from build123d import *

# Parameters (mm, degrees)
BOSS_EXTRUDE1_DEPTH = 19
SKETCH2_W           = 19
SKETCH2_H           = 80
BOSS_EXTRUDE2_DEPTH = 19
SKETCH3_W           = 19
SKETCH3_H           = 80
BOSS_EXTRUDE3_DEPTH = 19


with BuildPart() as part:
    # Sketch1 → Boss-Extrude1 (new body)
    with BuildSketch(Plane(origin=(0, 0, 0), x_dir=(0, 0, -1), z_dir=(1, 0, 0))):
        with BuildLine():
            Line((-143.772893773, 109.432234432), (-143.772893773, -140.567765568))
            Line((-143.772893773, -140.567765568), (96.227106227, -140.567765568))
            ThreePointArc((96.227106227, -140.567765568), (-42.958076814, -33.985541287), (-143.772893773, 109.432234432))
        make_face()
    extrude(amount=BOSS_EXTRUDE1_DEPTH)

    # Sketch2 → Boss-Extrude2 (add)
    with BuildSketch(Plane.XZ.offset(140.567765568)):
        with Locations((9.5, 23.772893773)):
            Rectangle(SKETCH2_W, SKETCH2_H)
    extrude(amount=BOSS_EXTRUDE2_DEPTH)

    # Sketch3 → Boss-Extrude3 (add)
    with BuildSketch(Plane.XY.offset(143.772893773)):
        with Locations((9.5, -20.567765568)):
            Rectangle(SKETCH3_W, SKETCH3_H)
    extrude(amount=BOSS_EXTRUDE3_DEPTH)


solid = part.part
CAD build for the part. Positions are in the model's coordinates, mm. A direction names the side the tool comes from. Round coordinates to 2 decimals unless told otherwise and drop trailing zeros. Order: outer loops, then holes, each group sorted by start corner. A loop starts at its lowest first (then second) coordinate and runs counter-clockwise, first axis right, second up. Notation, with made-up numbers: (18, 88.5) - (36, 88.5) arc R17 ccw to (36, 96.5) - close; hole circle Ø9 at (68.5, 20). An arc over 180 degrees is marked (long way). Return JSON: item names as keys, results as strings.
(1) Cut at A-A (x = 12.5). Give the cut face in (y, z).
Answer key:
{"outline": "(-159.57, -16.23) - (-140.57, -16.23) - (-140.57, -96.23) arc R577.79 cw to (109.43, 143.77) - (19.43, 143.77) - (19.43, 162.77) - (-60.57, 162.77) - (-60.57, 143.77) - (-140.57, 143.77) - (-140.57, 63.77) - (-159.57, 63.77) - close"}
(2) Tool access for faces 1 (the face through (9, 19.432, 153)), 2 (the face through (9, -140.568, -56)), 3 (the face through (9, -60.568, 153)), 4 (the face through (0, -64, 72)), 5 (the face through (9.37, -35.76, 41.25)): list every direction of +Z, -Z, +X, -X, +Y, -Y with a clear straight run to the whole face (end or side of a thin tool).
Answer key:
{"face 1": "+Z, +X, -X, +Y", "face 2": "-Z, +X, -X, -Y", "face 3": "+Z, +X, -X, -Y", "face 4": "+Z, -Z, -X, +Y, -Y", "face 5": "-Z, +X, -X, +Y"}
(3) Cut at C-C (z = 22.5). Give the cut face in (x, y), then the cut area to 3 significant figures.
Answer key:
{"outline": "(0, -159.57) - (19, -159.57) - (19, -54.26) - (0, -54.26) - close", "area": "2,000 mm^2"}
(4) Pin check, flat tips, straight feed: pin 1 Ø1.5 at (x, z) = (15, 23.5) entering from +Y; pin 2 Ø8 at (x, y) = (4, 15) entering from -Z; pin 3 Ø4 at (x, y) = (11.5, 32.5) entering from -Z. Stop position of each tip, or through.
Answer key:
{"pin 1": "stops at y = -52.6", "pin 2": "stops at z = 81.9", "pin 3": "stops at z = 96.44"}
(5) Wall check: probe 1 along Z at (x, y) = (11.5, -147.5); probe 2 along Y at (x, z) = (2.5, 118.5); probe 3 along Y at (x, z) = (1, -61.5). Give the ranges that are in metal, low to high. Write a range as from..to.
Answer key:
{"probe 1": "z = -16.23..63.77", "probe 2": "y = -140.57..63.78", "probe 3": "y = -140.57..-119.93"}
(6) Cut at B-B (y = 93). Give the cut face in (x, z), then the cut area to 3 significant figures.
Answer key:
{"outline": "(0, 135.29) - (19, 135.29) - (19, 143.77) - (0, 143.77) - close", "area": "161 mm^2"}
